Verification items for this drawing (mm, ordinates from the low corner). Coordinates: 2 decimals unless noted, no trailing zeros. Order: outer loops, then holes, each group sorted by start corner. A loop starts at its lowest first (then second) coordinate and runs counter-clockwise, first axis right, second up.
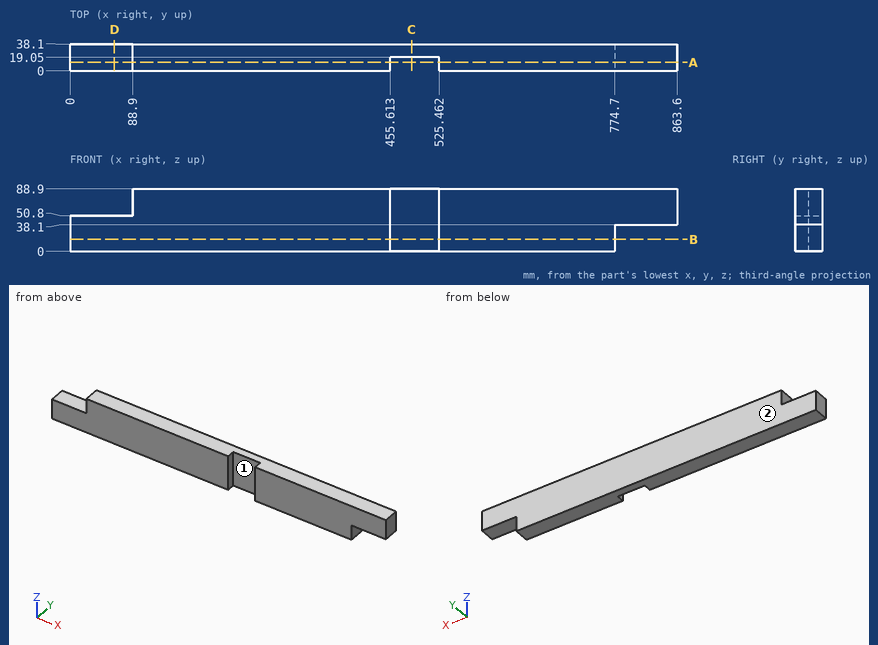
(1) Cross-section at D-D (x = 63). Enter the section's corners in (y, z).
Filled in:
outline: (0, 0) - (38.1, 0) - (38.1, 50.8) - (0, 50.8) - close
(2) Cross-section at C-C (x = 486). Enter the section's corners in (y, z).
Filled in:
outline: (19.05, 0) - (38.1, 0) - (38.1, 88.9) - (19.05, 88.9) - close
(3) Cross-section at A-A (y = 12). Enter the section's corners in (x, z).
Filled in:
outline: (0, 0) - (455.61, 0) - (455.61, 88.9) - (88.9, 88.9) - (88.9, 50.8) - (0, 50.8) - close; (525.46, 0) - (774.7, 0) - (774.7, 38.1) - (863.6, 38.1) - (863.6, 88.9) - (525.46, 88.9) - close
(4) Thickness scan on probe 1 along X at (y, z) = (15.5, 12); probe 2 along X at (y, z) = (10.5, 85.5); probe 3 along X at (y, z) = (32.5, 20). Record the ranges inside material, lowest first.
Filled in:
probe 1: x = 0 to 455.61, 525.46 to 774.7
probe 2: x = 88.9 to 455.61, 525.46 to 863.6
probe 3: x = 0 to 774.7
(5) Release check for a two-part mould opening along X. For the marked faces 1 and 2 record: +X half, -X half, draft (parallel to the pull), parting line (faces both ways), or undercut.
Filled in:
face 1: undercut
face 2: draft
(6) Cross-section at B-B (z = 17). Enter the section's corners in (x, y), and give its area (3 significant figures).
Filled in:
outline: (0, 0) - (455.61, 0) - (455.61, 19.05) - (525.46, 19.05) - (525.46, 0) - (774.7, 0) - (774.7, 38.1) - (0, 38.1) - close
area: 28,200 mm2
(7) Go/stop test with flat-tipped pins: P1, Ø19, axis at y = 11, z = 25.5, coming from the +X side; P2, Ø11.5, axis at x = 44.5, y = 20, coming from the +Z side; P3, Ø1.5, axis at y = 20, z = 37, coming from the -X side; P4, Ø19, axis at y = 15, z = 65, coming from the -X side. Record where each tip stops, or that it passes through.
Filled in:
P1: stops at x = 774.7
P2: stops at z = 50.8
P3: stops at x = 0
P4: stops at x = 88.9
